Source: CAD feature listing. Evaluate the final solid. Frame: model axes, mm. A direction names the side the tool comes from. Round coordinates to 2 decimals unless told otherwise and drop trailing zeros. Loops run counter-clockwise (first coordinate to the right, second up) from the corner with the lowest first, then second, coordinate; pieces in that order, holes last. Notation, with made-up numbers: (1.5, 21.25) - (58.5, 21.25) arc R9 cw to (58.5, 30.25) - close; hole circle Ø5 at (-10, -6.5). An arc over 180 degrees is marked (long way). Write item = value, one per line. Start each with the question number.
from build123d import *

# Parameters (mm, degrees)
F1_DEPTH  = 60
F2_DEPTH  = 5
F3_R      = 15
F4_DEPTH  = 8
F5_R      = 1.5
F6_DEPTH  = 68.001
F7_R      = 15
F8_DEPTH  = 4
F9_R      = 0.6
F11_DEPTH = 72.001


# Not quite as in the source:
# - a fillet or chamfer that OpenCascade refuses, or shapes differently, is made with other operations: its cross-section is extruded or revolved along the edge and cut away or added


with BuildPart() as f1:
    # F0 (on Top) → F1 (new body)
    with BuildSketch(Plane.XY):
        with BuildLine():
            ThreePointArc((4.344342247, 12.2526197379), (9.8886206176, 8.4389088324), (12.7832510794, 2.3639991203))
            ThreePointArc((12.7832510794, 2.3639991203), (13.8829504808, 1.9165651298), (14.9372441283, 1.3706705849))
            ThreePointArc((14.9372441283, 1.3706705849), (11.4099468664, 9.7372024989), (3.7020104756, 14.5359938923))
            ThreePointArc((3.7020104756, 14.5359938923), (4.0753636897, 13.4089875362), (4.344342247, 12.2526197379))
        make_face()
        with BuildLine():
            ThreePointArc((12.7832510794, 2.3639991203), (12.9456993637, 1.1869574482), (13, 0))
            ThreePointArc((13, 0), (12.6914373848, -2.8155669247), (11.7803973681, -5.4974755888))
            ThreePointArc((11.7803973681, -5.4974755888), (12.9572055714, -5.3404456491), (14.1147802532, -5.0767094072))
            ThreePointArc((14.1147802532, -5.0767094072), (14.7770379948, -2.5766544396), (15, 0))
            ThreePointArc((15, 0), (14.9843028187, 0.6860532326), (14.9372441283, 1.3706705849))
            ThreePointArc((14.9372441283, 1.3706705849), (13.8829504808, 1.9165651298), (12.7832510794, 2.3639991203))
        make_face()
        with BuildLine():
            ThreePointArc((14.1147802532, -5.0767094072), (12.9572055714, -5.3404456491), (11.7803973681, -5.4974755888))
            ThreePointArc((11.7803973681, -5.4974755888), (7.453385593, -10.6511522007), (1.1292451674, -12.9508611819))
            ThreePointArc((1.1292451674, -12.9508611819), (0.5785791746, -14.0026705342), (-0.0657478246, -14.9998559068))
            ThreePointArc((-0.0657478246, -14.9998559068), (8.6000602997, -12.2897910008), (14.1147802532, -5.0767094072))
        make_face()
        with BuildLine():
            ThreePointArc((-0.0657478246, -14.9998559068), (0.5785791746, -14.0026705342), (1.1292451674, -12.9508611819))
            ThreePointArc((1.1292451674, -12.9508611819), (-1.6450220625, -12.8954993084), (-4.344342247, -12.2526197379))
            ThreePointArc((-4.344342247, -12.2526197379), (-4.0753636897, -13.4089875362), (-3.7020104756, -14.5359938923))
            ThreePointArc((-3.7020104756, -14.5359938923), (-1.8981023799, -14.879422279), (-0.0657478246, -14.9998559068))
        make_face()
        with BuildLine():
            ThreePointArc((-3.7020104756, -14.5359938923), (-4.0753636897, -13.4089875362), (-4.344342247, -12.2526197379))
            ThreePointArc((-4.344342247, -12.2526197379), (-9.8886206176, -8.4389088324), (-12.7832510794, -2.3639991203))
            ThreePointArc((-12.7832510794, -2.3639991203), (-13.8829504808, -1.9165651298), (-14.9372441283, -1.3706705849))
            ThreePointArc((-14.9372441283, -1.3706705849), (-11.4099468664, -9.7372024989), (-3.7020104756, -14.5359938923))
        make_face()
        with BuildLine():
            ThreePointArc((-12.7832510794, -2.3639991203), (-12.8954993084, 1.6450220625), (-11.7803973681, 5.4974755888))
            ThreePointArc((-11.7803973681, 5.4974755888), (-12.9572055714, 5.3404456491), (-14.1147802532, 5.0767094072))
            ThreePointArc((-14.1147802532, 5.0767094072), (-14.879422279, 1.8981023799), (-14.9372441283, -1.3706705849))
            ThreePointArc((-14.9372441283, -1.3706705849), (-13.8829504808, -1.9165651298), (-12.7832510794, -2.3639991203))
        make_face()
        with BuildLine():
            ThreePointArc((-11.7803973681, 5.4974755888), (-7.453385593, 10.6511522007), (-1.1292451674, 12.9508611819))
            ThreePointArc((-1.1292451674, 12.9508611819), (-0.5785791746, 14.0026705342), (0.0657478246, 14.9998559068))
            ThreePointArc((0.0657478246, 14.9998559068), (-8.6000602997, 12.2897910008), (-14.1147802532, 5.0767094072))
            ThreePointArc((-14.1147802532, 5.0767094072), (-12.9572055714, 5.3404456491), (-11.7803973681, 5.4974755888))
        make_face()
        with BuildLine():
            ThreePointArc((-1.1292451674, 12.9508611819), (1.6450220625, 12.8954993084), (4.344342247, 12.2526197379))
            ThreePointArc((4.344342247, 12.2526197379), (4.0753636897, 13.4089875362), (3.7020104756, 14.5359938923))
            ThreePointArc((3.7020104756, 14.5359938923), (1.8981023799, 14.879422279), (0.0657478246, 14.9998559068))
            ThreePointArc((0.0657478246, 14.9998559068), (-0.5785791746, 14.0026705342), (-1.1292451674, 12.9508611819))
        make_face()
    extrude(amount=F1_DEPTH)

    # F0 (on Top) → F2 (join)
    with BuildSketch(Plane.XY):
        with BuildLine():
            ThreePointArc((3.7020104756, 14.5359938923), (11.4099468664, 9.7372024989), (14.9372441283, 1.3706705849))
            ThreePointArc((14.9372441283, 1.3706705849), (17.2222714986, -0.3046475231), (19.0900610331, -2.4352350245))
            ThreePointArc((19.0900610331, -2.4352350245), (22.4559354435, 2.0084712145), (23.6511522007, 7.453385593))
            ThreePointArc((23.6511522007, 7.453385593), (16.0960665792, 19.2581688359), (2.2122433682, 17.3420062106))
            ThreePointArc((2.2122433682, 17.3420062106), (3.0431666419, 15.9846802304), (3.7020104756, 14.5359938923))
        make_face()
        with BuildLine():
            ThreePointArc((19.0900610331, -2.4352350245), (17.2222714986, -0.3046475231), (14.9372441283, 1.3706705849))
            ThreePointArc((14.9372441283, 1.3706705849), (14.9843028187, 0.6860532326), (15, 0))
            ThreePointArc((15, 0), (14.7770379948, -2.5766544396), (14.1147802532, -5.0767094072))
            ThreePointArc((14.1147802532, -5.0767094072), (16.7472118135, -4.0286898812), (19.0900610331, -2.4352350245))
        make_face()
        with BuildLine():
            ThreePointArc((19.0900610331, -2.4352350245), (16.7472118135, -4.0286898812), (14.1147802532, -5.0767094072))
            ThreePointArc((14.1147802532, -5.0767094072), (8.6000602997, -12.2897910008), (-0.0657478246, -14.9998559068))
            ThreePointArc((-0.0657478246, -14.9998559068), (-1.0671791062, -16.2367482592), (-2.2122433682, -17.3420062106))
            ThreePointArc((-2.2122433682, -17.3420062106), (12.346275042, -22.2875112657), (21.4389088324, -9.8886206176))
            ThreePointArc((21.4389088324, -9.8886206176), (20.8377994805, -5.981254408), (19.0900610331, -2.4352350245))
        make_face()
        with BuildLine():
            ThreePointArc((0.0657478246, 14.9998559068), (1.8981023799, 14.879422279), (3.7020104756, 14.5359938923))
            ThreePointArc((3.7020104756, 14.5359938923), (3.0431666419, 15.9846802304), (2.2122433682, 17.3420062106))
            ThreePointArc((2.2122433682, 17.3420062106), (1.0671791062, 16.2367482592), (0.0657478246, 14.9998559068))
        make_face()
        with BuildLine():
            ThreePointArc((-2.2122433682, -17.3420062106), (-1.0671791062, -16.2367482592), (-0.0657478246, -14.9998559068))
            ThreePointArc((-0.0657478246, -14.9998559068), (-1.8981023799, -14.879422279), (-3.7020104756, -14.5359938923))
            ThreePointArc((-3.7020104756, -14.5359938923), (-3.0431666419, -15.9846802304), (-2.2122433682, -17.3420062106))
        make_face()
        with BuildLine():
            ThreePointArc((-14.1147802532, 5.0767094072), (-8.6000602997, 12.2897910008), (0.0657478246, 14.9998559068))
            ThreePointArc((0.0657478246, 14.9998559068), (1.0671791062, 16.2367482592), (2.2122433682, 17.3420062106))
            ThreePointArc((2.2122433682, 17.3420062106), (-15.8922944255, 20.5397728182), (-19.0900610331, 2.4352350245))
            ThreePointArc((-19.0900610331, 2.4352350245), (-16.7472118135, 4.0286898812), (-14.1147802532, 5.0767094072))
        make_face()
        with BuildLine():
            ThreePointArc((-2.2122433682, -17.3420062106), (-3.0431666419, -15.9846802304), (-3.7020104756, -14.5359938923))
            ThreePointArc((-3.7020104756, -14.5359938923), (-11.4099468664, -9.7372024989), (-14.9372441283, -1.3706705849))
            ThreePointArc((-14.9372441283, -1.3706705849), (-17.2222714986, 0.3046475231), (-19.0900610331, 2.4352350245))
            ThreePointArc((-19.0900610331, 2.4352350245), (-20.5397728182, -15.8922944255), (-2.2122433682, -17.3420062106))
        make_face()
        with BuildLine():
            ThreePointArc((-14.9372441283, -1.3706705849), (-14.879422279, 1.8981023799), (-14.1147802532, 5.0767094072))
            ThreePointArc((-14.1147802532, 5.0767094072), (-16.7472118135, 4.0286898812), (-19.0900610331, 2.4352350245))
            ThreePointArc((-19.0900610331, 2.4352350245), (-17.2222714986, 0.3046475231), (-14.9372441283, -1.3706705849))
        make_face()
    extrude(amount=F2_DEPTH)

    # F3 (on face) → F4 (join)
    with BuildSketch(Plane.XY.offset(60)):
        Circle(F3_R)
    extrude(amount=F4_DEPTH)

    # F5 (on face) → F6 (cut, through all)
    with BuildSketch(Plane.XY.offset(68)):
        Circle(F5_R)
    extrude(amount=-F6_DEPTH, mode=Mode.SUBTRACT)

    # F7 (on face) → F8 (join)
    with BuildSketch(Plane.XY.offset(68)):
        Circle(F7_R)
    extrude(amount=F8_DEPTH)

    # F10: fillet of radius 7 on 1 edges, made by hand

    # F10_s1 → F10_t2 (revolve, cut)
    with BuildSketch(Plane.XZ):
        with BuildLine():
            ThreePointArc((15, 65), (12.9497474683, 69.9497474683), (8, 72))
            Line((8, 72), (15, 72))
            Line((15, 72), (15, 65))
        make_face()
    revolve(axis=Axis((0, 0, 72), (0, 0, 1)), mode=Mode.SUBTRACT)

    # F9 (on face) → F11 (cut, through all)
    with BuildSketch(Plane.XY.offset(72)):
        Circle(F9_R)
    extrude(amount=-F11_DEPTH, mode=Mode.SUBTRACT)


solid = f1.part
(1) Material intervals for line 1 along Y through (x, z) = (0.5, 18.5); line 2 along Y through (x, z) = (0, 62), sorted ascending. Write a range as from..to.
(2) Pin query (flat end, axial travel): P1, Ø3, axis at x = 6, z = 51.5, coming from the +Y side; P2, Ø12, axis at x = 4.5, z = 64.5, coming from the -Y side; P3, Ø1.8, axis at x = 0, y = 0, coming from the +Z side; P4, Ø5, axis at x = -9.5, z = 32.5, coming from the -Y side. Return the tip coordinate at first contact, or that it passes through.
(3) Cut plane B-B (z = 46). Output: boundary loops of the cut face in (x, y).
(4) Cut plane C-C (x = 17.5). Output: boundary loops of the cut face in (y, z), and give its area (3 significant figures).
(5) Access query for faces 1 (the face through (15.4, 0.3, 5)), 2 (the face through (3, 0, 60)), 3 (the face through (-20.7, -15.7, 2.5)). Directions: +Z, -Z, +X, -X, +Y, -Y. A direction counts if a zero-diameter tool reaches every point of the face in a straight line with its end or side. Return the directions, or none.
(6) Mould query, pull axis X, two halves, no side actions, for faces 4 (the face through (10, -10, 0)), 5 (the face through (12.97, -7.536, 34.58)), 6 (the face through (1, 0, 68)). Classes: +X half, -X half, draft (parallel to the pull), parting line (faces both ways), or undercut.
(7) Cut plane A-A (y = 18.5). Output: boundary loops of the cut face in (x, z), and give its area (3 significant figures).
Solution:
q1.line_1 = -14.99..-12.99, 12.99..14.99
q1.line_2 = -15..-1.5, 1.5..15
q2.P1 = 14.31
q2.P2 = -15
q2.P3 = 72
q2.P4 = -13.27
q3.outline = circle Ø30 at (0, 0); hole circle Ø26 at (0, 0)
q4.outline = (-19.21, 0) - (18.5, 0) - (18.5, 5) - (-19.21, 5) - close
q4.area = 189 mm^2
q5.face_1 = +Z
q5.face_2 = -Z
q5.face_3 = +Z, -Z
q6.face_4 = draft
q6.face_5 = parting line
q6.face_6 = undercut
q7.outline = (-18.18, 0) - (1.3, 0) - (1.3, 5) - (-18.18, 5) - close; (3.8, 0) - (17.5, 0) - (17.5, 5) - (3.8, 5) - close
q7.area = 166 mm^2
